Design review of the part built by this model. Coordinates are the model's own, in mm. Round coordinates to 2 decimals unless told otherwise and drop trailing zeros. Loops run counter-clockwise (first coordinate to the right, second up) from the corner with the lowest first, then second, coordinate; pieces in that order, holes last. Notation, with made-up numbers: (80, -12.5) -> (91, -12.5) arc R19 cw to (91, 18.5) -> close; hole circle Ø10 at (-28.75, 76.5). An arc over 180 degrees is marked (long way). Write each question's results on one line, items separated by ' | '. Start each with the question number.
from build123d import *

# Parameters (mm, degrees)
SKETCH1_W           = 609.6
SKETCH1_H           = 609.6
BOSS_EXTRUDE1_DEPTH = 6.35
CUT_EXTRUDE2_DEPTH  = 432.099063441
SKETCH4_W           = 25.4
SKETCH4_H           = 25.4
CUT_EXTRUDE8_DEPTH  = 432.099063441
FILLET4_R           = 12.7
FILLET5_R           = 12.7
SKETCH5_R           = 3.175
CUT_EXTRUDE9_DEPTH  = 432.099063441


with BuildPart() as part:
    # Sketch1 → Boss-Extrude1 (new body)
    with BuildSketch(Plane(origin=(0, 0, 0), x_dir=(1, 0, 0), z_dir=(0, 1, 0))):
        Rectangle(SKETCH1_W, SKETCH1_H)
    extrude(amount=BOSS_EXTRUDE1_DEPTH)

    # Sketch3 → Cut-Extrude2 (cut, through all)
    with BuildSketch(Plane(origin=(0, 0, 0), x_dir=(1, 0, 0), z_dir=(0, 1, 0))):
        with BuildLine():
            Line((-3.175, 193.254689298), (-3.175, 142.454689298))
            ThreePointArc((-3.175, 142.454689298), (-45.125573361, 120.304111538), (-50.492310608, 73.169232396))
            ThreePointArc((-50.492310608, 73.169232396), (-76.989658396, 44.45), (-88.612569335, 7.143007484))
            ThreePointArc((-88.612569335, 7.143007484), (-126.749203452, -21.072162878), (-124.95687982, -68.477713992))
            Line((-124.95687982, -68.477713992), (-168.950970332, -93.877713992))
            Line((-168.950970332, -93.877713992), (-173.656481646, -98.42752932))
            Line((-173.656481646, -98.42752932), (-176.009237303, -100.702436985))
            Line((-176.009237303, -100.702436985), (-179.308794092, -102.607436985))
            ThreePointArc((-179.308794092, -102.607436985), (-179.599326756, -103.691719649), (-178.515044092, -103.982252313))
            Line((-178.515044092, -103.982252313), (-175.215487303, -102.077252313))
            Line((-175.215487303, -102.077252313), (-172.068981646, -101.177159977))
            Line((-172.068981646, -101.177159977), (-165.775970332, -99.376975306))
            Line((-165.775970332, -99.376975306), (-121.78187982, -73.976975306))
            ThreePointArc((-121.78187982, -73.976975306), (-81.623630091, -99.23194866), (-38.120258727, -80.31223988))
            ThreePointArc((-38.120258727, -80.31223988), (0, -88.9), (38.120258727, -80.31223988))
            ThreePointArc((38.120258727, -80.31223988), (81.623630091, -99.23194866), (121.78187982, -73.976975306))
            Line((121.78187982, -73.976975306), (165.775970332, -99.376975306))
            Line((165.775970332, -99.376975306), (172.068981646, -101.177159977))
            Line((172.068981646, -101.177159977), (175.215487303, -102.077252313))
            Line((175.215487303, -102.077252313), (178.515044092, -103.982252313))
            ThreePointArc((178.515044092, -103.982252313), (179.599326756, -103.691719649), (179.308794092, -102.607436985))
            Line((179.308794092, -102.607436985), (176.009237303, -100.702436985))
            Line((176.009237303, -100.702436985), (173.656481646, -98.42752932))
            Line((173.656481646, -98.42752932), (168.950970332, -93.877713992))
            Line((168.950970332, -93.877713992), (124.95687982, -68.477713992))
            ThreePointArc((124.95687982, -68.477713992), (126.749203452, -21.072162878), (88.612569335, 7.143007484))
            ThreePointArc((88.612569335, 7.143007484), (76.989658396, 44.45), (50.492310608, 73.169232396))
            ThreePointArc((50.492310608, 73.169232396), (45.125573361, 120.304111538), (3.175, 142.454689298))
            Line((3.175, 142.454689298), (3.175, 193.254689298))
            Line((3.175, 193.254689298), (1.5875, 199.604689298))
            Line((1.5875, 199.604689298), (0.79375, 202.779689298))
            Line((0.79375, 202.779689298), (0.79375, 206.589689298))
            ThreePointArc((0.79375, 206.589689298), (0, 207.383439298), (-0.79375, 206.589689298))
            Line((-0.79375, 206.589689298), (-0.79375, 202.779689298))
            Line((-0.79375, 202.779689298), (-1.5875, 199.604689298))
            Line((-1.5875, 199.604689298), (-3.175, 193.254689298))
        make_face()
    extrude(amount=CUT_EXTRUDE2_DEPTH, mode=Mode.SUBTRACT)

    # Sketch4 → Cut-Extrude8 (cut, through all)
    with BuildSketch(Plane(origin=(0, 0, 0), x_dir=(1, 0, 0), z_dir=(0, 1, 0))):
        with Locations((12.7, -190.5)):
            Rectangle(SKETCH4_W, SKETCH4_H)
        with Locations((-190.5, 12.7)):
            Rectangle(SKETCH4_W, SKETCH4_H)
    extrude(amount=CUT_EXTRUDE8_DEPTH, mode=Mode.SUBTRACT)

    # Fillet4
    fillet4_edges = [part.edges().sort_by_distance(p)[0] for p in [
        (-177.8, 3.175, -25.4),
    ]]
    fillet(fillet4_edges, radius=FILLET4_R)

    # Fillet5
    fillet5_edges = [part.edges().sort_by_distance(p)[0] for p in [
        (25.4, 3.175, 177.8),
    ]]
    fillet(fillet5_edges, radius=FILLET5_R)

    # Sketch5 → Cut-Extrude9 (cut, through all)
    with BuildSketch(Plane(origin=(0, 6.35, 0), x_dir=(1, 0, 0), z_dir=(0, 1, 0))):
        with Locations(Location((-254, 254, 0), (0, 0, 270))):
            Circle(SKETCH5_R)
        with Locations(Location((254, 254, 0), (0, 0, 270))):
            Circle(SKETCH5_R)
        with Locations(Location((254, -254, 0), (0, 0, 270))):
            Circle(SKETCH5_R)
        with Locations(Location((-254, -254, 0), (0, 0, 270))):
            Circle(SKETCH5_R)
    extrude(amount=-CUT_EXTRUDE9_DEPTH, mode=Mode.SUBTRACT)


solid = part.part
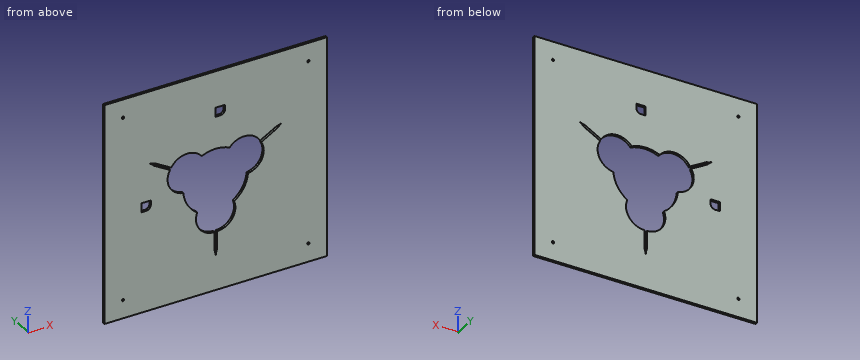
1) Take a section at C-C (y = 3.25). State how many separate pieces and enclosed holes the cut face has, plus the area to 3 significant figures.
2) Take a section at B-B (z = -47.5). Write out the cut boundary in (x, y), plus the area to 3 significant figures.
3) To check wall thickness, follow line 1 (X direction, y = 2.25, z = -254) (3 decimals); line 2 (X direction, y = 5, z = -165) (3 decimals). State the ranges of each line that lie inside material, in increasing order. Write a range as from..to.
4) Insertion check: pin 1 (5 mm diameter, centred on x = 254, z = -254, fed in from +Y). The pin has a flat end and moves straight along its axis. Give the tip position at first contact, or say it passes through.
5) Take a section at A-A (x = 102). Write out the cut boundary in (y, z).
Geometry check:
1) separate pieces: 1 | enclosed holes: 7 | area: 329,000 mm^2
2) outline: (-304.8, 0) -> (-75.15, 0) -> (-75.15, 6.35) -> (-304.8, 6.35) -> close; (75.15, 0) -> (304.8, 0) -> (304.8, 6.35) -> (75.15, 6.35) -> close | area: 2,920 mm^2
3) line 1: x = -304.8..-257.175, -250.825..250.825, 257.175..304.8 | line 2: x = -304.8..-3.175, 3.175..304.8
4) pin 1: passes through
5) outline: (0, -304.8) -> (6.35, -304.8) -> (6.35, -3.16) -> (0, -3.16) -> close; (0, 93.24) -> (6.35, 93.24) -> (6.35, 304.8) -> (0, 304.8) -> close
